from build123d import *

# Parameters (mm, degrees)
F1_DEPTH = 63.5
F3_D     = 12.7
F4_D     = 12.7


with BuildPart() as f1:
    # F0 (on Front) → F1 (new body)
    with BuildSketch(Plane.XZ):
        Polygon((-38.1, -12.7), (-38.1, 0), (38.1, 0), (38.1, -12.7), (57.15, -12.7), (57.15, 22.225), (22.225, 22.225), (22.225, 34.925), (-22.225, 34.925), (-22.225, 22.225), (-57.15, 22.225), (-57.15, -12.7), align=None)
    extrude(amount=F1_DEPTH)

    # F3 (through all)
    with Locations(Plane(origin=(0, 0, 0), x_dir=(1, 0, 0), z_dir=(0, 0, -1))):
        with Locations((0, 47.625)):
            Hole(F3_D / 2)

    # F4 (through all)
    with Locations(Plane(origin=(0, 0, 0), x_dir=(1, 0, 0), z_dir=(0, 0, -1))):
        with Locations((0, 15.875)):
            Hole(F4_D / 2)


solid = f1.part
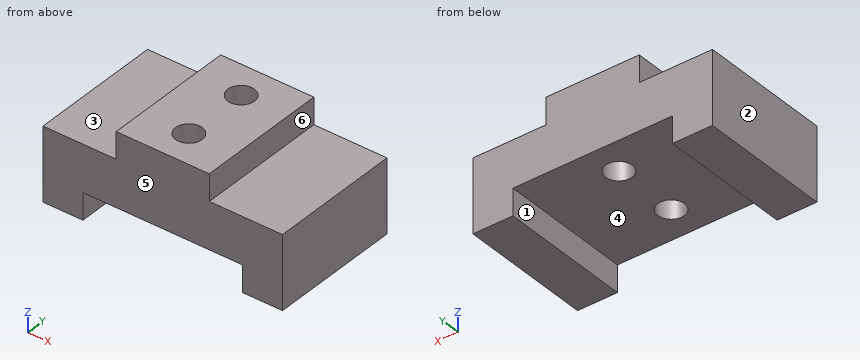
Check sheet for the modelled part. Datum: model origin and axes. Units: mm. Face numbers are marked on the shaded views. A direction names the side the tool comes from. Give positions to 0.01 mm unless a question says otherwise; leave off trailing zeros. Order: outer loops, then holes, each group sorted by start corner. A loop starts at its lowest first (then second) coordinate and runs counter-clockwise, first axis right, second up. Notation, with made-up numbers: M -36.75,60 L -28.75,60 A9 ccw -28.75,69 Z; hole C 88,66.5 d10. An arc over 180 degrees is marked long. Answer as CSV lines item,"result". Start each with the question number.
Item 1: Tool access check on the marked faces 4, 5 and 6. Record the directions out of +Z, -Z, +X, -X, +Y, -Y that give a thin tool (end or side, any length) a straight path to the whole face; none if there is none.
Item 2: Cross-section at A-A on z = -3.5. Enter the section's corners in (x, y).
Item 3: Gauge pin test, flat ends, axial feed: P1, Ø14, axis at y = -36.5, z = 28, coming from the +X side; P2, Ø17.5, axis at x = -46, y = -34, coming from the +Z side (3 decimals); P3, Ø3, axis at y = -23.5, z = 28.5, coming from the +X side (3 decimals); P4, Ø19, axis at x = 3.5, y = -37, coming from the -Z side. Record the tip position at first contact, or that the pin passes through.
Item 4: Thickness scan on line 1 (Y direction, x = 0, z = 12) (3 decimals); line 2 (X direction, y = -19.5, z = -7); line 3 (Z direction, x = 26, y = -17) (3 decimals). Record the ranges inside material, lowest first. Write a range as [from, to].
Item 5: Mould release check, pull along X, two halves, no side actions. Record for the marked faces 1, 2 and 3: +X half, -X half, draft (parallel to the pull), parting line (faces both ways), or undercut.
Item 6: Cross-section at B-B on x = 0. Enter the section's corners in (y, z) (3 decimals).
Item 7: Cross-section at C-C on y = -32.5. Enter the section's corners in (x, z) (3 decimals), plus the area to 3 significant figures.
Item 8: Cross-section at D-D on y = -11. Enter the section's corners in (x, z) (3 decimals).
Established:
1,face 4,"-Z, +Y, -Y"
1,face 5,"+Z, -Z, +X, -X, -Y"
1,face 6,"+Z, +X, +Y, -Y"
2,outline,"M -57.15,-63.5 L -38.1,-63.5 L -38.1,0 L -57.15,0 Z; M 38.1,-63.5 L 57.15,-63.5 L 57.15,0 L 38.1,0 Z"
3,P1,"stops at x = 57.15"
3,P2,"stops at z = 22.225"
3,P3,"stops at x = 22.225"
3,P4,"stops at z = 0"
4,line 1,"y = [-63.5, -53.975], [-41.275, -22.225], [-9.525, 0]"
4,line 2,"x = [-57.15, -38.1], [38.1, 57.15]"
4,line 3,"z = [0, 22.225]"
5,face 1,"undercut"
5,face 2,"-X half"
5,face 3,"draft"
6,outline,"M -63.5,0 L -53.975,0 L -53.975,34.925 L -63.5,34.925 Z; M -41.275,0 L -22.225,0 L -22.225,34.925 L -41.275,34.925 Z; M -9.525,0 L 0,0 L 0,34.925 L -9.525,34.925 Z"
7,outline,"M -57.15,-12.7 L -38.1,-12.7 L -38.1,0 L 38.1,0 L 38.1,-12.7 L 57.15,-12.7 L 57.15,22.225 L 22.225,22.225 L 22.225,34.925 L -22.225,34.925 L -22.225,22.225 L -57.15,22.225 Z"
7,area,"3,590 mm^2"
8,outline,"M -57.15,-12.7 L -38.1,-12.7 L -38.1,0 L -4.069,0 L -4.069,34.925 L -22.225,34.925 L -22.225,22.225 L -57.15,22.225 Z; M 4.069,0 L 38.1,0 L 38.1,-12.7 L 57.15,-12.7 L 57.15,22.225 L 22.225,22.225 L 22.225,34.925 L 4.069,34.925 Z"
